Check sheet for the modelled part. Datum: model origin and axes. Units: mm. Face numbers are marked on the shaded views. A direction names the side the tool comes from. Give positions to 0.01 mm unless a question says otherwise; leave off trailing zeros. Loops run counter-clockwise (first coordinate to the right, second up) from the corner with the lowest first, then second, coordinate; pieces in that order, holes last.
```python
from build123d import *

# Parameters (mm, degrees)
DODANIE_WYCI_GNI_CIE1_DEPTH    = 60
OTWORY_USTALAJ_CE_1_0MM1_D     = 11
OTWORY_USTALAJ_CE_1_0MM1_DEPTH = 22.25
OTWORY_USTALAJ_CE_1_0MM1_TIP   = 3.304733405
OTW_R_GWINTOWANY_M51_D         = 4.2
OTW_R_GWINTOWANY_M51_DEPTH     = 14
OTW_R_GWINTOWANY_M51_TIP       = 1.2618073
ZAOKR_GLENIE1_R                = 0.5
SFAZOWANIE3_SIZE               = 0.5


with BuildPart() as part:
    # Szkic1 → Dodanie-wyciągnięcie1 (new body)
    with BuildSketch(Plane.XY):
        Polygon((0, 3), (0, 53), (3, 53), (3, 3), (40, 3), (40, 0), (0, 0), align=None)
    extrude(amount=DODANIE_WYCI_GNI_CIE1_DEPTH)

    # Otwory ustalające Ø1.0mm1
    with Locations(Plane(origin=(0, 3, 0), x_dir=(1, 0, 0), z_dir=(0, 1, 0))):
        with Locations((20, -45), (20, -15)):
            Hole(OTWORY_USTALAJ_CE_1_0MM1_D / 2, depth=OTWORY_USTALAJ_CE_1_0MM1_DEPTH)
            with Locations((0, 0, -(OTWORY_USTALAJ_CE_1_0MM1_DEPTH + OTWORY_USTALAJ_CE_1_0MM1_TIP / 2))):  # 118° drill point
                Cone(0, OTWORY_USTALAJ_CE_1_0MM1_D / 2, OTWORY_USTALAJ_CE_1_0MM1_TIP, mode=Mode.SUBTRACT)

    # Otwór gwintowany M51
    with Locations(Plane(origin=(3, 0, 0), x_dir=(0, 0, -1), z_dir=(1, 0, 0))):
        with Locations((-50, 45), (-40, 33), (-30, 45), (-20, 33), (-10, 45)):
            Hole(OTW_R_GWINTOWANY_M51_D / 2, depth=OTW_R_GWINTOWANY_M51_DEPTH)
            with Locations((0, 0, -(OTW_R_GWINTOWANY_M51_DEPTH + OTW_R_GWINTOWANY_M51_TIP / 2))):  # 118° drill point
                Cone(0, OTW_R_GWINTOWANY_M51_D / 2, OTW_R_GWINTOWANY_M51_TIP, mode=Mode.SUBTRACT)

    # Zaokrąglenie1
    zaokr_glenie1_edges = [part.edges().sort_by_distance(p)[0] for p in [
        (3, 3, 30),
    ]]
    fillet(zaokr_glenie1_edges, radius=ZAOKR_GLENIE1_R)

    # Sfazowanie3
    sfazowanie3_edges = [part.edges().sort_by_distance(p)[0] for p in [
        (0, 53, 30),
        (3, 53, 30),
        (40, 1.5, 60),
        (40, 3, 30),
        (40, 0, 30),
        (0, 0, 30),
        (21.75, 3, 60),
        (1.5, 53, 60),
        (0, 26.5, 60),
        (3, 28.25, 0),
        (3, 28.25, 60),
        (3.146446609, 3.146446609, 0),
        (3.146446609, 3.146446609, 60),
        (0, 26.5, 0),
        (1.5, 53, 0),
        (21.75, 3, 0),
        (20, 0, 60),
        (40, 1.5, 0),
        (20, 0, 0),
    ]]
    chamfer(sfazowanie3_edges, length=SFAZOWANIE3_SIZE)


solid = part.part
```
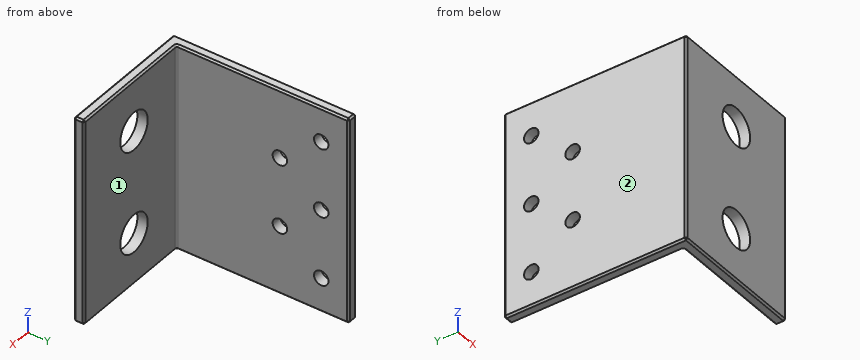
(1) Section check D-D on x = 32. Record the boundary of the cut face in (y, z).
(2) Section check A-A on z = 45. Record the boundary of the cut face in (x, y).
(3) Material ranges on line 1 (Z direction, x = 20, y = 2); line 2 (Y direction, x = 1, z = 40); line 3 (X direction, y = 36, z = 24), recorded low to high.
(4) Gauge pin test, flat ends, axial feed: pin 1 Ø4 at (y, z) = (45, 30) entering from +X; pin 2 Ø3 at (y, z) = (34, 26.5) entering from -X; pin 3 Ø4 at (y, z) = (28.5, 31) entering from +X; pin 4 Ø1 at (x, z) = (6, 7) entering from +Y. Record the tip position at first contact, or that the pin passes through.
(5) Access from +Z, -Z, +X, -X, +Y, -Y to the whole of each face (thin tool, end or side, straight path). Record for the marked faces 1 and 2.
(6) Section check B-B on x = 20. Record the boundary of the cut face in (y, z), plus the area to 4 significant figures.
(7) Section check C-C on y = 45. Record the boundary of the cut face in (x, z), plus the area to 3 significant figures.
Computed values:
1. outline: (0, 0.5) - (0.5, 0) - (2.5, 0) - (3, 0.5) - (3, 59.5) - (2.5, 60) - (0.5, 60) - (0, 59.5) - close
2. outline: (0, 0.5) - (0.5, 0) - (14.5, 0) - (14.5, 3) - (3.5, 3) arc R0.5 cw to (3, 3.5) - (3, 52.5) - (2.5, 53) - (0.5, 53) - (0, 52.5) - close; (25.5, 0) - (39.5, 0) - (40, 0.5) - (40, 2.5) - (39.5, 3) - (25.5, 3) - close
3. line 1: z = 0 to 9.5, 20.5 to 39.5, 50.5 to 60
3. line 2: y = 0 to 30.9, 35.1 to 53
3. line 3: x = 0 to 3
4. pin 1: passes through
4. pin 2: stops at x = 0
4. pin 3: stops at x = 3
4. pin 4: stops at y = 3
5. face 1: +Z, -Z, +X, +Y
5. face 2: +Z, -Z, -X, +Y, -Y
6. outline: (0, 0.5) - (0.5, 0) - (2.5, 0) - (3, 0.5) - (3, 9.5) - (0, 9.5) - close; (0, 20.5) - (3, 20.5) - (3, 39.5) - (0, 39.5) - close; (0, 50.5) - (3, 50.5) - (3, 59.5) - (2.5, 60) - (0.5, 60) - (0, 59.5) - close
6. area: 113.5 mm2
7. outline: (0, 0.5) - (0.5, 0) - (2.5, 0) - (3, 0.5) - (3, 7.9) - (0, 7.9) - close; (0, 12.1) - (3, 12.1) - (3, 27.9) - (0, 27.9) - close; (0, 32.1) - (3, 32.1) - (3, 47.9) - (0, 47.9) - close; (0, 52.1) - (3, 52.1) - (3, 59.5) - (2.5, 60) - (0.5, 60) - (0, 59.5) - close
7. area: 142 mm2
